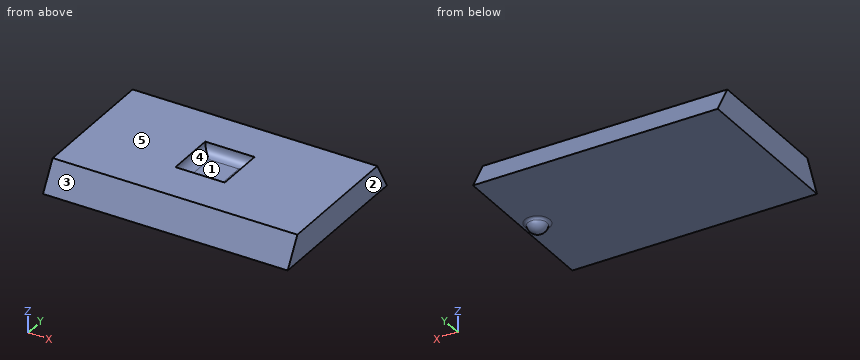
Autodesk Inventor part; units mm, degrees
ref_plane "Work Plane1" through (1.5, 8.5, 2.9) normal (1, 0, 0) x (0, 1, 0)
ref_plane "Work Plane2" through (23.3, 8.5, 0.1) normal (-1, 0, 0) x (0, -1, 0)
ref_plane "YZ Plane" through (0, 0, 0) normal (1, 0, 0) x (0, 1, 0)
sketch "Sketch1" plane through (0, 0, 0) normal (1, 0, 0) x (0, 1, 0)
  line L0 (0, 0) -> (1.7321, 3) construction
  line L1 (1.7321, 3) -> (15.2679, 3) construction
  line L2 (15.2679, 3) -> (17, 0) construction
  line L3 (17, 0) -> (0, 0) construction
  line L4 (15.2679, 3) -> (15.2679, 0) construction
  line L5 (0.1732, 0.1) -> (1.7898, 2.9)
  line L6 (1.7898, 2.9) -> (15.2102, 2.9)
  line L7 (15.2102, 2.9) -> (16.8268, 0.1)
  line L8 (16.8268, 0.1) -> (0.1732, 0.1)
  line L9 (16.0185, 1.5) -> (16.1051, 1.55) construction
  dimension "d0" = 60
  dimension "d1" = 17
  dimension "d2" = 3
  dimension "d11" = 0.1
extrude "Extrusion1" add sketch "Sketch1" along normal blind 24.8
sketch "Sketch3" plane through (0, 1.7898, 2.9) normal (0, 0, 1) x (1, 0, 0)
  line L0 (0, 13.4204) -> (0, 0) construction
  line L1 (0, 13.4204) -> (24.8, 13.4204) construction
  line L2 (0, 0) -> (3, 0) construction
  line L3 (3, 0) -> (3, 13.4204) construction
  line L4 (3, 13.4204) -> (0, 13.4204) construction
  line L5 (0, 13.4204) -> (0, 0) construction
  circle A0 centre (1.5, 6.7102) radius 1.0891
  line L6 (0, 6.7102) -> (3, 6.7102) construction
  point P0 (0, -1.7898)
  point P1 (1.5, 13.4204)
  dimension "d12" = 3
ref_plane "Work Plane1" through (1.5, 8.5, 2.9) normal (1, 0, 0) x (0, 1, 0)
sketch "Sketch5" plane through (0, 0.1732, 0.1) normal (0, 0, -1) x (-1, 0, 0)
  line L0 (0, 0) -> (0, 16.6536) construction
  line L1 (0, 16.6536) -> (-24.8, 16.6536) construction
  line L2 (-24.8, 0) -> (-24.8, 16.6536) construction
  line L3 (0, 0) -> (-24.8, 0) construction
  line L4 (-21.8, 0) -> (-21.8, 16.6536) construction
  line L5 (-24.8, 8.3268) -> (-21.8, 8.3268) construction
  point P0 (0, -0.1732)
  point P1 (-23.3, 8.3268)
  dimension "d16" = 3
ref_plane "Work Plane2" through (23.3, 8.5, 0.1) normal (-1, 0, 0) x (0, -1, 0)
sketch "Sketch6" plane through (23.3, 8.5, 0.1) normal (-1, 0, 0) x (0, -1, 0)
  line L0 (8.3268, 0) -> (-8.3268, 0)
  line L1 (0, 0) -> (0, -1)
  line L2 (0, 0) -> (-1, 0)
  arc A0 (-1, 0) -> (0, -1) centre (0, 0) ccw
  point P0 (8.5, -0.1)
  dimension "d17" = 1
revolve "Revolution2" add sketch "Sketch6" angle 360 about axis through (23.3, 8.5, 0.1) along (0, 0, -1)
fillet "Fillet4" radius 0.3 1 edges at (23.3, 7.5, 0.1)
sketch "Sketch7" plane through (0, 1.7898, 2.9) normal (0, 0, 1) x (1, 0, 0)
  line L0 (9.9, 4.2102) -> (14.9, 4.2102)
  line L1 (14.9, 4.2102) -> (14.9, 9.2102)
  line L2 (14.9, 9.2102) -> (9.9, 9.2102)
  line L3 (9.9, 9.2102) -> (9.9, 4.2102)
  line L4 (0, 13.4204) -> (0, 0)
  line L5 (0, 13.4204) -> (24.8, 13.4204)
  point P0 (0, -1.7898)
  point P1 (9.9, 6.7102)
  point P2 (0, 6.7102)
  point P3 (12.4, 9.2102)
  point P4 (12.4, 13.4204)
  dimension "d20" = 5
  dimension "d21" = 5
extrude "Extrusion3" cut sketch "Sketch7" against normal blind 1
fillet "Fillet5" radius 1 4 edges at (9.9, 8.5, 1.9) (12.4, 6, 1.9) (14.9, 8.5, 1.9) (12.4, 11, 1.9)
properties part number "door"
Source: CAD feature listing. Evaluate the final solid. Frame: model axes, mm. Face numbers are marked on the shaded views. A direction names the side the tool comes from. Round coordinates to 2 decimals unless told otherwise and drop trailing zeros. Loops run counter-clockwise (first coordinate to the right, second up) from the corner with the lowest first, then second, coordinate; pieces in that order, holes last. Notation, with made-up numbers: M 17,59.25 L 47,59.25 A29 ccw 47,94.25 Z; hole C -30,16 d10. An arc over 180 degrees is marked long. Answer as CSV lines item,"result".
Q1. Line query: line 1 along Z through (x, y) = (15, 7.75); line 2 along Z through (x, y) = (2.5, 16); line 3 along Y through (x, z) = (3.5, 1.7). Output: solid intervals per line, ascending.
Verdict:
line 1,"z = 0.1 to 2.9"
line 2,"z = 0.1 to 1.53"
line 3,"y = 1.1 to 15.9"
Q2. Contact query for flat-ended pins moving along their axis: pin 1 (1.5 mm diameter, centred on x = 12, y = 8.5, fed in from +Z); pin 2 (5 mm diameter, centred on x = 10.5, y = 9, fed in from -Z); pin 3 (1.5 mm diameter, centred on x = 18, z = 0.5, fed in from -Y); pin 4 (2 mm diameter, centred on y = 14, z = 2, fed in from -X). Output: stop coordinate, or through.
Verdict:
pin 1,"stops at z = 1.9"
pin 2,"stops at z = 0.1"
pin 3,"stops at y = 0.17"
pin 4,"stops at x = 0"
Q3. Reachability of the marked faces 1 and 2 from +Z, -Z, +X, -X, +Y, -Y: full face, straight path, thin tool, end or side. Return the list, or none.
Verdict:
face 1,"+Z"
face 2,"+Z, -Z, +X, +Y, -Y"
Q4. Pull-direction query (Y, two-part tool) for the marked faces 3, 4 and 5; classes: +Y half, -Y half, draft (parallel to the pull), parting line (faces both ways), or undercut.
Verdict:
face 3,"-Y half"
face 4,"undercut"
face 5,"draft"
Q5. Cut plane B-B (x = 18.25). Return the cut outline in (y, z), plus the area to 3 significant figures.
Verdict:
outline,"M 0.17,0.1 L 16.83,0.1 L 15.21,2.9 L 1.79,2.9 Z"
area,"42.1 mm^2"
Q6. Cut plane D-D (z = -0.4). Return the cut outline in (x, y), plus the area to 3 significant figures.
Verdict:
outline,"C 23.3,8.5 d1.73"
area,"2.36 mm^2"
Q7. Cut plane A-A (z = 2.3). Return the cut outline in (x, y).
Verdict:
outline,"M 0,1.44 L 24.8,1.44 L 24.8,15.56 L 0,15.56 Z; hole M 10.1,6.2 L 14.7,6.2 L 14.7,10.8 L 10.1,10.8 Z"
Q8. Cut plane C-C (y = 15.5). Return the cut outline in (x, z), plus the area to 3 significant figures.
Verdict:
outline,"M 0,0.1 L 24.8,0.1 L 24.8,2.4 L 0,2.4 Z"
area,"57.0 mm^2"
